from build123d import *

# Parameters (mm, degrees)
SKETCH1_W           = 10
SKETCH1_H           = 13
SKETCH1_R           = 0.8
BOSS_EXTRUDE1_DEPTH = 5
CUT_EXTRUDE2_DEPTH  = 3.5
SKETCH4_R           = 1.25
CUT_EXTRUDE3_DEPTH  = 7.5
SKETCH5_R           = 0.95
CUT_EXTRUDE4_DEPTH  = 3


with BuildPart() as part:
    # Sketch1 → Boss-Extrude1 (new body)
    with BuildSketch(Plane.XY):
        Rectangle(SKETCH1_W, SKETCH1_H)
        with Locations((0, 3)):
            Circle(SKETCH1_R, mode=Mode.SUBTRACT)
    extrude(amount=BOSS_EXTRUDE1_DEPTH)

    # Sketch3 → Cut-Extrude2 (cut)
    with BuildSketch(Plane.ZY.offset(5)):
        with BuildLine():
            Line((-1.6, -3.5), (-1.6, -7.6))
            Line((-1.6, -7.6), (6.6, -7.6))
            Line((6.6, -7.6), (6.6, -3.5))
            ThreePointArc((6.6, -3.5), (2.5, 0.6), (-1.6, -3.5))
        make_face()
    cut_extrude2 = extrude(amount=-CUT_EXTRUDE2_DEPTH, mode=Mode.SUBTRACT)

    # Mirror1: Cut-Extrude2 across plane
    add(cut_extrude2.mirror(Plane(origin=(0, 0, 0), x_dir=(0, 0, 1), z_dir=(1, 0, 0))), mode=Mode.SUBTRACT)

    # Sketch4 → Cut-Extrude3 (cut, through all)
    with BuildSketch(Plane.ZY.offset(1.5)):
        with Locations((2.5, -3.5)):
            Circle(SKETCH4_R)
    extrude(amount=-CUT_EXTRUDE3_DEPTH, mode=Mode.SUBTRACT)

    # Sketch5 → Cut-Extrude4 (cut)
    with BuildSketch(Plane(origin=(0, 6.5, 0), x_dir=(1, 0, 0), z_dir=(0, 1, 0))):
        with Locations((0, -2.5)):
            Circle(SKETCH5_R)
    extrude(amount=-CUT_EXTRUDE4_DEPTH, mode=Mode.SUBTRACT)


solid = part.part
Geometry: final body of the model. Coordinates: model frame, mm. A direction names the side the tool comes from. Give positions to 0.01 mm unless a question says otherwise; leave off trailing zeros. Write each loop counter-clockwise with the first axis right and the second up, starting at its lowest first coordinate (ties: lowest second). Pieces come first, ordered by that corner, then holes.
(1) Access query for faces 1 (the cylindrical face through (0.9, 5, 2.2)), 2 (the cylindrical face through (3.3, 0.6, 2.5)), 3 (the cylindrical face through (-3.3, 0.6, 2.5)). Directions: +Z, -Z, +X, -X, +Y, -Y. A direction counts if a zero-diameter tool reaches every point of the face in a straight line with its end or side. Return the directions, or none.
(2) Mould query, pull axis Y, two halves, no side actions, for faces 4 (the flat face through (1.5, -2, 2)), 5 (the flat face through (0, -6.5, 2)), 6 (the cylindrical face through (-0.021, -3.979, 3.655)), 7 (the cylindrical face through (-0.17, 2.22, 2.46)). Classes: released by +Y, released by -Y, zero draft, split by the parting line, or undercut.
(3) First-contact query: P1, Ø2, axis at y = -0.5, z = 3, coming from the -X side; P2, Ø2.5, axis at y = -2.5, z = 1.5, coming from the +X side. Flat tips, straight axial feed; report the tip coordinate or a pass-through.
(4) Cut plane D-D, the plane z = 1. Return loops of the section in (x, y), then the cut area to 3 significant figures.
(5) Cut plane B-B, the plane y = -3.5. Return loops of the section in (x, z), then the cut area to 3 significant figures.
(6) Cut plane A-A, the plane x = 0. Return loops of the section in (y, z).
(7) Ray query, line 1 (Z direction, x = 0, y = 5.6); line 2 (Y direction, x = 0, z = 3.95); line 3 (X direction, y = 3.75, z = 2.45). Return the intervals inside material, ascending.
(8) Cut plane C-C, the plane z = 2.5. Return loops of the section in (x, y).
Values follow:
1. face 1: +Y
1. face 2: +X, -Y
1. face 3: -X, -Y
2. face 4: zero draft
2. face 5: released by -Y
2. face 6: undercut
2. face 7: undercut
3. P1: stops at x = -1.5
3. P2: stops at x = 1.5
4. outline: (-5, 0.32) - (-1.5, 0.32) - (-1.5, -6.5) - (1.5, -6.5) - (1.5, 0.32) - (5, 0.32) - (5, 6.5) - (-5, 6.5) - close; hole circle Ø1.6 at (0, 3)
4. area: 80.3 mm2
5. outline: (-1.5, 0) - (1.5, 0) - (1.5, 1.25) - (-1.5, 1.25) - close; (-1.5, 3.75) - (1.5, 3.75) - (1.5, 5) - (-1.5, 5) - close
5. area: 7.50 mm2
6. outline: (-6.5, 0) - (2.2, 0) - (2.2, 5) - (-6.5, 5) - close; (3.8, 0) - (6.5, 0) - (6.5, 1.55) - (3.8, 1.55) - close; (3.8, 3.45) - (6.5, 3.45) - (6.5, 5) - (3.8, 5) - close; hole circle Ø2.5 at (-3.5, 2.5)
7. line 1: z = 0 to 1.55, 3.45 to 5
7. line 2: y = -6.5 to 2.2, 3.8 to 6.5
7. line 3: x = -5 to -0.95, 0.95 to 5
8. outline: (-5, 0.6) - (-1.5, 0.6) - (-1.5, -2.25) - (1.5, -2.25) - (1.5, 0.6) - (5, 0.6) - (5, 6.5) - (0.95, 6.5) - (0.95, 3.5) - (0.62, 3.5) arc R0.8 cw (long way) to (-0.62, 3.5) - (-0.95, 3.5) - (-0.95, 6.5) - (-5, 6.5) - close; (-1.5, -6.5) - (1.5, -6.5) - (1.5, -4.75) - (-1.5, -4.75) - close
